```python
from build123d import *

# Parameters (mm, degrees)
F0_W     = 66.675
F0_H     = 76.2
F0_R     = 6.35
F1_DEPTH = 9.525
F2_W     = 66.675
F2_H     = 76.2
F3_DEPTH = 3.175
F5_DEPTH = 3.175
F6_R     = 1.5875


with BuildPart() as f1:
    # F0 (on Top) → F1 (new body)
    with BuildSketch(Plane.XY):
        Rectangle(F0_W, F0_H)
        with BuildLine():
            Line((60.325, 38.1), (33.3375, 38.1))
            Line((33.3375, 38.1), (33.3375, -38.1))
            Line((33.3375, -38.1), (60.325, -38.1))
            ThreePointArc((60.325, -38.1), (69.305256, -34.380256), (73.025, -25.4))
            Line((73.025, -25.4), (73.025, 25.4))
            ThreePointArc((73.025, 25.4), (69.305256, 34.380256), (60.325, 38.1))
        make_face()
        with Locations((60.325, -25.4)):
            Circle(F0_R, mode=Mode.SUBTRACT)
        with Locations((60.325, 25.4)):
            Circle(F0_R, mode=Mode.SUBTRACT)
        with BuildLine():
            Line((-33.3375, 38.1), (-60.325, 38.1))
            ThreePointArc((-60.325, 38.1), (-69.305256, 34.380256), (-73.025, 25.4))
            Line((-73.025, 25.4), (-73.025, -25.4))
            ThreePointArc((-73.025, -25.4), (-69.305256, -34.380256), (-60.325, -38.1))
            Line((-60.325, -38.1), (-33.3375, -38.1))
            Line((-33.3375, -38.1), (-33.3375, 38.1))
        make_face()
        with Locations((-60.325, -25.4)):
            Circle(F0_R, mode=Mode.SUBTRACT)
        with Locations((-60.325, 25.4)):
            Circle(F0_R, mode=Mode.SUBTRACT)
    extrude(amount=F1_DEPTH)

    # F2 (on face) → F3 (join)
    with BuildSketch(Plane.XY.offset(9.525)):
        Rectangle(F2_W, F2_H)
    extrude(amount=F3_DEPTH)

    # F4 (on face) → F5 (cut)
    with BuildSketch(Plane(origin=(0, 0, 0), x_dir=(1, 0, 0), z_dir=(0, 0, -1))):
        Polygon((33.3375, -38.1), (33.3375, 38.1), (-32.625852, 38.1), (-34.035566, -38.1), align=None)
    extrude(amount=-F5_DEPTH, mode=Mode.SUBTRACT)

    # F6
    f6_edges = [f1.edges().sort_by_distance(p)[0] for p in [
        (33.3375, 0, 3.175),
        (-33.330709, 0, 3.175),
    ]]
    fillet(f6_edges, radius=F6_R)


solid = f1.part
```
Source: CAD feature listing. Evaluate the final solid. Frame: model axes, mm. A direction names the side the tool comes from. Give positions to 0.01 mm unless a question says otherwise; leave off trailing zeros. Write each loop counter-clockwise with the first axis right and the second up, starting at its lowest first coordinate (ties: lowest second). Pieces come first, ordered by that corner, then holes. Notation, with made-up numbers: (71, 74) - (120, 74) arc R13 cw to (120, 94) - close; hole circle Ø9 at (58.25, -7). An arc over 180 degrees is marked (long way). One line per item, written item: value. Start each with the question number.
Q1. Section query A-A, the plane z = 7.75. Return the cut outline in (x, y) (3 decimals), then the cut area to 3 significant figures.
Q2. First-contact query: pin 1 Ø7.5 at (x, y) = (60.325, -25.4) entering from +Z; pin 2 Ø20 at (x, y) = (48, -16.5) entering from +Z (3 decimals); pin 3 Ø3.5 at (y, z) = (18, 11.5) entering from -X; pin 4 Ø1.5 at (x, y) = (-9, -9.5) entering from -Z (3 decimals). Flat tips, straight axial feed; report the tip coordinate or a pass-through.
Q3. Section query B-B, the plane x = 41.5. Return the cut outline in (y, z) (3 decimals), then the cut area to 3 significant figures.
Q4. Draft query along X for faces 1 (the face through (-53, 1, 0)), 2 (the face through (-54.46, -27.83, 4.7)), 3 (the face through (-69.206, 34.478, 4.696)). Return one class per face: +X half, -X half, draft (parallel to the pull), parting line (faces both ways), or undercut.
Q5. Material intervals for probe 1 along Y at (x, z) = (-61, 7.5); probe 2 along X at (y, z) = (-21.5, 1) (1 decimal); probe 3 along Z at (x, y) = (-3, -3.5) (3 decimals), sorted ascending. Write a range as from..to.
Q6. Set-up query: faces 4 (the face through (-33.338, -1, 11)), 5 (the face through (-32.888, 0.527, 2.698)), 6 (the face through (53, 1, 0)), 7 (the face through (53, 1, 9.525)). Return all of +Z, -Z, +X, -X, +Y, -Y with unobstructed straight access to the full face (end or side cutting, diameter ignored); none if empty.
Answer:
1. outline: (-73.025, -25.4) arc R12.7 ccw to (-60.325, -38.1) - (60.325, -38.1) arc R12.7 ccw to (73.025, -25.4) - (73.025, 25.4) arc R12.7 ccw to (60.325, 38.1) - (-60.325, 38.1) arc R12.7 ccw to (-73.025, 25.4) - close; hole circle Ø12.7 at (-60.325, -25.4); hole circle Ø12.7 at (-60.325, 25.4); hole circle Ø12.7 at (60.325, -25.4); hole circle Ø12.7 at (60.325, 25.4)
1. area: 10,500 mm2
2. pin 1: passes through
2. pin 2: stops at z = 9.525
2. pin 3: stops at x = -33.34
2. pin 4: stops at z = 3.175
3. outline: (-38.1, 0) - (38.1, 0) - (38.1, 9.525) - (-38.1, 9.525) - close
3. area: 726 mm2
4. face 1: draft
4. face 2: undercut
4. face 3: -X half
5. probe 1: y = -38.08..-31.71, -19.09..19.09, 31.71..38.08
5. probe 2: x = -73..-65.3, -55.3..-32.9, 33.3..55.3, 65.3..73
5. probe 3: z = 3.175..12.7
6. face 4: +Z, -X, +Y, -Y
6. face 5: -Z, +Y
6. face 6: -Z, +X, -X, +Y, -Y
6. face 7: +Z, +X, +Y, -Y
